For this review, take the finished solid that the model builds, in its own axes (mm). A direction names the side the tool comes from. Coordinates: 2 decimals unless noted, no trailing zeros. Write each loop counter-clockwise with the first axis right and the second up, starting at its lowest first coordinate (ties: lowest second). Pieces come first, ordered by that corner, then holes.
```python
from build123d import *

# Parameters (mm, degrees)
SKETCH_1_W          = 68
SKETCH_1_H          = 12
EXTRUDE_1_DEPTH     = 38
SKETCH_3_R          = 1.5
SKETCH_3_R_2        = 5
CUT_EXTRUDE_1_DEPTH = 3
FILLET_1_R          = 4


with BuildPart() as part:
    # Эскиз1 → Повернуть1 (revolve)
    with BuildSketch(Plane(origin=(0, 0, 0), x_dir=(0, 0, -1), z_dir=(1, 0, 0)), mode=Mode.PRIVATE) as revolve_1_sk:
        with Locations((34, 6)):
            Rectangle(SKETCH_1_W, SKETCH_1_H)
        Polygon((68, 12), (68, 0), (94, 0), (94, 34), (68, 34), align=None)
    revolve(revolve_1_sk.sketch.rotate(Axis((0, 0, 0), (0, 0, -1)), 90), axis=Axis((0, 0, 0), (0, 0, -1)))

    # Эскиз2 → Бобышка-Вытянуть1 (add)
    with BuildSketch(Plane.XY.offset(-68)):
        Polygon((0, 21), (13, 21), (13, 18), (-13, 18), (-13, 21), align=None)
    extrude(amount=EXTRUDE_1_DEPTH)

    # Эскиз3 → Вырез-Вытянуть1 (cut)
    with BuildSketch(Plane(origin=(0, 21, 0), x_dir=(1, 0, 0), z_dir=(0, 1, 0))):
        with Locations(Location((-7.7, 51.1, 0), (0, 0, 270))):
            Circle(SKETCH_3_R)
        with Locations(Location((7.7, 51.1, 0), (0, 0, 270))):
            Circle(SKETCH_3_R)
        with Locations(Location((7.7, 37.5, 0), (0, 0, 270))):
            Circle(SKETCH_3_R)
        with Locations(Location((-7.7, 37.5, 0), (0, 0, 270))):
            Circle(SKETCH_3_R)
        with Locations(Location((0, 44.3, 0), (0, 0, 270))):
            Circle(SKETCH_3_R_2)
    extrude(amount=-CUT_EXTRUDE_1_DEPTH, mode=Mode.SUBTRACT)

    # Скругление1
    fillet_1_edges = [part.edges().sort_by_distance(p)[0] for p in [
        (-13, 19.5, -30),
        (13, 19.5, -30),
    ]]
    fillet(fillet_1_edges, radius=FILLET_1_R)


solid = part.part
```
Q1. Add section B-B (z = -44.3). State the section outline as (x, y) points, then the cut area to 3 significant figures.
Ans:
outline: (-13, 18) - (-5, 18) - (-5, 21) - (-13, 21) - close; circle Ø24 at (0, 0); (5, 18) - (13, 18) - (13, 21) - (5, 21) - close
area: 500 mm2
Q2. Draft analysis for pull direction Z (two halves, no side actions). For faces 1 (the cylindrical face through (-6.69, 19.52, -38.61)), 2 (the flat face through (0, 0, 0)), 3 (the flat face through (0, 0, -94)), state which applies: +Z half, -Z half, draft (parallel to the pull), parting line (faces both ways), or undercut.
Ans:
face 1: undercut
face 2: +Z half
face 3: -Z half
Q3. Add section D-D (y = 0). State the section outline as (x, z) points.
Ans:
outline: (-34, -94) - (34, -94) - (34, -68) - (12, -68) - (12, 0) - (-12, 0) - (-12, -68) - (-34, -68) - close
Q4. Add section A-A (z = -66.5). State the section outline as (x, y) points.
Ans:
outline: (-13, 18) - (13, 18) - (13, 21) - (-13, 21) - close; circle Ø24 at (0, 0)
Q5. Clearance check with flat-ended pins moving along their axes: pin 1 Ø1.5 at (y, z) = (19.5, -52.5) entering from -X; pin 2 Ø2 at (x, y) = (-11, -19) entering from +Z; pin 3 Ø4 at (y, z) = (-10.5, -78) entering from -X. State where each tip first meets the part, or that it passes through.
Ans:
pin 1: stops at x = -13
pin 2: stops at z = -68
pin 3: stops at x = -32.92
Q6. Add section C-C (x = 7.7). State the section outline as (y, z) points.
Ans:
outline: (-33.12, -94) - (33.12, -94) - (33.12, -68) - (21, -68) - (21, -52.6) - (18, -52.6) - (18, -68) - (9.2, -68) - (9.2, 0) - (-9.2, 0) - (-9.2, -68) - (-33.12, -68) - close; (18, -49.6) - (21, -49.6) - (21, -39) - (18, -39) - close; (18, -36) - (21, -36) - (21, -30) - (18, -30) - close
Q7. Tool access review of faces 4 (the flat face through (3, 21, -49)), 5 (the cylindrical face through (-11.859, 19.521, -31.203)), 6 (the cylindrical face through (-8.275, 19.521, -49.714)): name each direction out of +Z, -Z, +X, -X, +Y, -Y from which nothing blocks a thin tool from reaching the whole face with its end or side.
Ans:
face 4: +Z, +X, -X, +Y
face 5: +Z, -X, +Y
face 6: +Y
Q8. For probe 1 along X at (y, z) = (18.6, -51.1); probe 2 along Z at (x, y) = (7, 20); probe 3 along X at (y, z) = (20, -50.5), list the stretches that pass through material, from the lowest coordinate up.
Ans:
probe 1: x = -13 to -9.2, -6.2 to 6.2, 9.2 to 13
probe 2: z = -94 to -52.43, -49.77 to -38.83, -36.17 to -30
probe 3: x = -13 to -9.07, -6.33 to 6.33, 9.07 to 13
